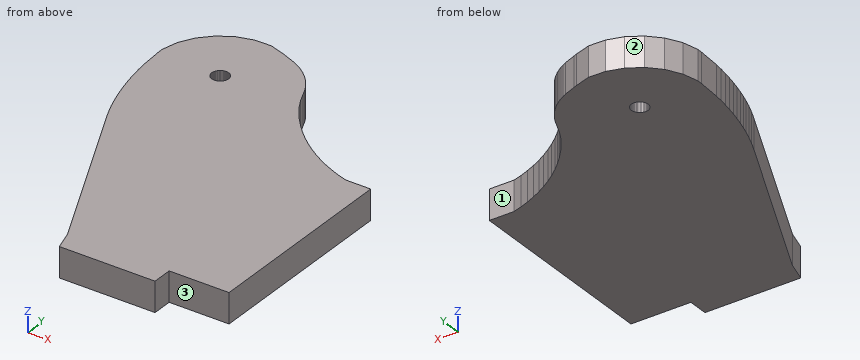
```python
from build123d import *

# Parameters (mm, degrees)
F1_DEPTH = 3


with BuildPart() as f1:
    # F0 (on Top) → F1 (new body)
    with BuildSketch(Plane.XY):
        Polygon((2.510942, 9.469501), (2.373605, 9.605645), (1.790243, 10.337165), (1.153897, 11.268456), (0.607543, 12.255246), (0.155931, 13.288848), (-0.011836, 13.688085), (-0.205334, 14.075512), (-0.423774, 14.44945), (-0.666191, 14.808327), (-0.931545, 15.150541), (-1.218717, 15.474696), (-1.526489, 15.779394), (-1.853514, 16.06329), (-2.198395, 16.32519), (-2.559685, 16.563975), (-2.935808, 16.77863), (-3.325165, 16.968241), (-4.495444, 17.43362), (-4.835398, 17.568824), (-6.383731, 18.062981), (-8.041005, 18.025669), (-9.632137, 17.560696), (-11.048721, 16.699738), (-12.194184, 15.501493), (-12.9905, 14.047597), (-13.383387, 12.437161), (-13.371246, 11.897258), (-13.221005, 9.551822), (-13.127761, 8.77377), (-13.01308, 7.998612), (-12.876987, 7.226884), (-12.719634, 6.459245), (-12.541148, 5.696229), (-12.341606, 4.938446), (-12.12121, 4.186453), (-11.880139, 3.440862), (-11.618519, 2.702204), (-11.229289, 1.746326), (-10.804017, 0.805917), (-2.786634, -16.062985), (-2.205609, -18.063007), (7.383374, -18.063007), (7.383374, -16.062985), (13.383387, -16.062985), (13.383387, 4.095013), (11.383391, 4.095013), (10.88964, 4.095013), (9.997161, 4.375937), (9.121089, 4.704512), (8.263992, 5.079771), (7.428357, 5.500675), (6.616573, 5.965927), (5.831053, 6.474257), (5.074031, 7.024116), (4.347693, 7.61398), (3.654196, 8.242071), (2.995549, 8.906612), align=None)
        Polygon((-6.247359, 11.961622), (-6.227369, 11.856771), (-6.220663, 11.750243), (-6.227369, 11.643716), (-6.247359, 11.538839), (-6.280353, 11.437341), (-6.325794, 11.340744), (-6.382995, 11.250625), (-6.451041, 11.16838), (-6.528841, 11.095304), (-6.615201, 11.032566), (-6.70875, 10.981131), (-6.807987, 10.941837), (-6.911391, 10.915294), (-7.017283, 10.901909), (-7.12404, 10.901909), (-7.229932, 10.915294), (-7.333336, 10.941837), (-7.432573, 10.981131), (-7.526122, 11.032566), (-7.612482, 11.095304), (-7.690282, 11.16838), (-7.758328, 11.250625), (-7.815529, 11.340744), (-7.86097, 11.437341), (-7.893964, 11.538839), (-7.913954, 11.643716), (-7.92066, 11.750243), (-7.913954, 11.856771), (-7.893964, 11.961622), (-7.86097, 12.063146), (-7.815529, 12.159717), (-7.758328, 12.249861), (-7.690282, 12.332106), (-7.612482, 12.405182), (-7.526122, 12.46792), (-7.432573, 12.51933), (-7.333336, 12.558624), (-7.229932, 12.585192), (-7.12404, 12.598552), (-7.017283, 12.598552), (-6.911391, 12.585192), (-6.807987, 12.558624), (-6.70875, 12.51933), (-6.615201, 12.46792), (-6.528841, 12.405182), (-6.451041, 12.332106), (-6.382995, 12.249861), (-6.325794, 12.159717), (-6.280353, 12.063146), align=None, mode=Mode.SUBTRACT)
    extrude(amount=F1_DEPTH)


solid = f1.part
```
Here's how the part is built. I have some questions about the finished solid (model axes, mm). Face numbers are marked on the shaded views. A direction names the side the tool comes from. Round coordinates to 2 decimals unless told otherwise and drop trailing zeros. Write each loop counter-clockwise with the first axis right and the second up, starting at its lowest first coordinate (ties: lowest second). Pieces come first, ordered by that corner, then holes.
Q1. Please list where these lines run through material, in increasing order: probe 1 along X at (y, z) = (-8, 1.8); probe 2 along Y at (x, z) = (8.25, 1.75); probe 3 along Y at (x, z) = (-1.25, 2.35).
Q2. If we section it at B-B on x = -9.25: Write out the boundary of the cut face in (y, z).
Q3. Will these pins go through, and if not, where does the flat tip stop? P1, Ø1.5, axis at x = -6, z = 1.5, coming from the -Y side; P2, Ø1, axis at x = 8.5, z = 1.5, coming from the +Y side; P3, Ø1, axis at y = -17.5, z = 2, coming from the +X side.
Q4. Which directions (+Z, -Z, +X, -X, +Y, -Y) give clear straight access to the entire face, cutting with the end or side of a thin tool? Please do the marked faces 1, 2 and 3.
Q5. If we section it at A-A on y = 0: Write out the boundary of the cut face in (x, z), plus the area to 3 significant figures.
Answer below:
1. probe 1: x = -6.62 to 13.38
1. probe 2: y = -16.06 to 5.09
1. probe 3: y = -18.06 to 15.51
2. outline: (-2.46, 0) - (17.67, 0) - (17.67, 3) - (-2.46, 3) - close
3. P1: stops at y = -10.88
3. P2: stops at y = 5.21
3. P3: stops at x = 7.38
4. face 1: +Z, -Z, +X, +Y
4. face 2: +Z, -Z, -X, +Y
4. face 3: +Z, -Z, +X, -Y
5. outline: (-10.42, 0) - (13.38, 0) - (13.38, 3) - (-10.42, 3) - close
5. area: 71.4 mm2
